```python
from build123d import *

# Parameters (mm, degrees)
F0_R      = 18.54
F1_DEPTH  = 15
F2_R      = 17.1
F3_DEPTH  = 11
F5_R      = 4.535
F6_DEPTH  = 6
F9_DEPTH  = 9.01
F7_R      = 4.535
F10_DEPTH = 1.5
F11_DEPTH = 3.4


with BuildPart() as f1:
    # F0 (on Front) → F1 (new body)
    with BuildSketch(Plane.XZ):
        Circle(F0_R)
        with BuildLine():
            ThreePointArc((-2.5, -3.7836787654), (-2.1481067245, 3.9939782799), (4.535, 0))
            ThreePointArc((4.535, 0), (3.9939782799, -2.1481067245), (2.5, -3.7836787654))
            ThreePointArc((2.5, -3.7836787654), (0, -4.535), (-2.5, -3.7836787654))
        make_face(mode=Mode.SUBTRACT)
        with BuildLine():
            ThreePointArc((2.5, -3.7836787654), (3.9939782799, -2.1481067245), (4.535, 0))
            ThreePointArc((4.535, 0), (-2.1481067245, 3.9939782799), (-2.5, -3.7836787654))
            Line((-2.5, -3.7836787654), (2.5, -3.7836787654))
        make_face()
        with BuildLine():
            Line((2.5, -3.7836787654), (-2.5, -3.7836787654))
            ThreePointArc((-2.5, -3.7836787654), (0, -4.535), (2.5, -3.7836787654))
        make_face()
    extrude(amount=F1_DEPTH)

    # F2 (on face) → F3 (cut)
    with BuildSketch(Plane.XZ.offset(15)):
        Circle(F2_R)
    extrude(amount=-F3_DEPTH, mode=Mode.SUBTRACT)

    # F5 (on face) → F6 (join)
    with BuildSketch(Plane.XZ.offset(4)):
        Circle(F5_R)
    extrude(amount=F6_DEPTH)

    # F8 (on face) → F9 (cut)
    with BuildSketch(Plane.XZ.offset(10)):
        with BuildLine():
            ThreePointArc((1.662322006, -3.4171165547), (3.221554254, -2.0153382318), (3.8, 0))
            ThreePointArc((3.8, 0), (-2.0153382318, 3.221554254), (-1.662322006, -3.4171165547))
            Line((-1.662322006, -3.4171165547), (1.662322006, -3.4171165547))
        make_face()
    extrude(amount=-F9_DEPTH, mode=Mode.SUBTRACT)

    # F7 (on face) → F10 (join)
    with BuildSketch(Plane.XZ.offset(10)):
        Circle(F7_R)
    extrude(amount=F10_DEPTH)

    # F11 (cut): a face of the model
    f11_faces = [f1.faces().sort_by_distance(p)[0] for p in [
        (0, -11.5, 0),
    ]]
    extrude(f11_faces, amount=-F11_DEPTH, mode=Mode.SUBTRACT)


solid = f1.part
```
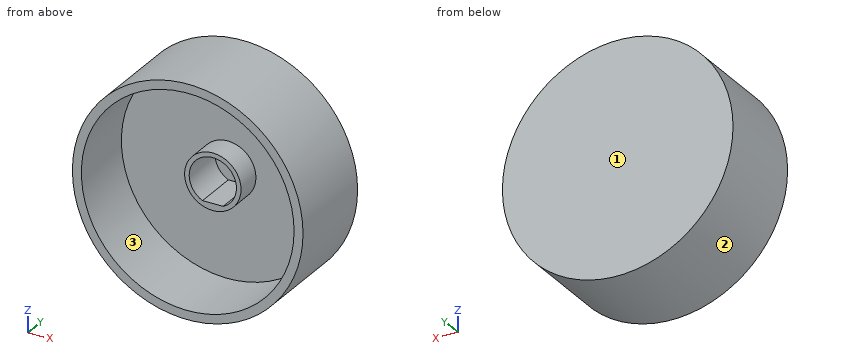
Design review of the part built by this model. Coordinates are the model's own, in mm. Face numbers are marked on the shaded views. Coordinates: 2 decimals unless noted, no trailing zeros. Order: outer loops, then holes, each group sorted by start corner. A loop starts at its lowest first (then second) coordinate and runs counter-clockwise, first axis right, second up.
1) Wall thickness on line 1 along Z through (x, y) = (0, -5.75) (3 decimals); line 2 along Z through (x, y) = (0, -12.5); line 3 along Z through (x, y) = (0, -2): over which ranges is each line inside the solid? List them lowest first.
2) Take a section at A-A, the plane y = -6. Give the boundary of the cut face in (x, z) (3 decimals).
3) Take a section at D-D, the plane y = -9.75. Give the boundary of the cut face in (x, z).
4) Clearance check with flat-ended pins moving along their axes: pin 1 (8.5 mm diameter, centred on x = 0, z = 0, fed in from -Y); pin 2 (2 mm diameter, centred on x = 7.5, z = 6, fed in from -Y); pin 3 (2 mm diameter, centred on x = 1, z = 0, fed in from -Y). State where each tip first meets the part, or that it passes through.
5) Take a section at C-C, the plane x = 0. Give the boundary of the cut face in (y, z) (3 decimals).
6) Mouldability with a two-part tool opening along Z and no side actions: class the marked faces 1, 2 and 3 as +Z half, -Z half, draft (parallel to the pull), parting line (faces both ways), or undercut.
7) Take a section at B-B, the plane z = 0. Give the boundary of the cut face in (x, y) (3 decimals), and give its area (3 significant figures).
Returned:
1. line 1: z = -18.54 to -17.1, -4.535 to -3.417, 3.8 to 4.535, 17.1 to 18.54
1. line 2: z = -18.54 to -17.1, 17.1 to 18.54
1. line 3: z = -18.54 to -3.42, 3.8 to 18.54
2. outline: circle Ø37.08 at (0, 0); circle Ø9.07 at (0, 0); hole circle Ø34.2 at (0, 0); hole (-1.662, -3.417) - (1.662, -3.417) arc R3.8 ccw (long way) to start
3. outline: circle Ø37.08 at (0, 0); hole circle Ø34.2 at (0, 0)
4. pin 1: stops at y = -8.1
4. pin 2: stops at y = -4
4. pin 3: stops at y = -0.99
5. outline: (-15, -18.54) - (0, -18.54) - (0, 18.54) - (-15, 18.54) - (-15, 17.1) - (-4, 17.1) - (-4, 4.535) - (-8.1, 4.535) - (-8.1, 3.8) - (-0.99, 3.8) - (-0.99, -3.417) - (-8.1, -3.417) - (-8.1, -4.535) - (-4, -4.535) - (-4, -17.1) - (-15, -17.1) - close
6. face 1: draft
6. face 2: parting line
6. face 3: undercut
7. outline: (-18.54, -15) - (-17.1, -15) - (-17.1, -4) - (-4.535, -4) - (-4.535, -8.1) - (-3.8, -8.1) - (-3.8, -0.99) - (3.8, -0.99) - (3.8, -8.1) - (4.535, -8.1) - (4.535, -4) - (17.1, -4) - (17.1, -15) - (18.54, -15) - (18.54, 0) - (-18.54, 0) - close
7. area: 163 mm2
